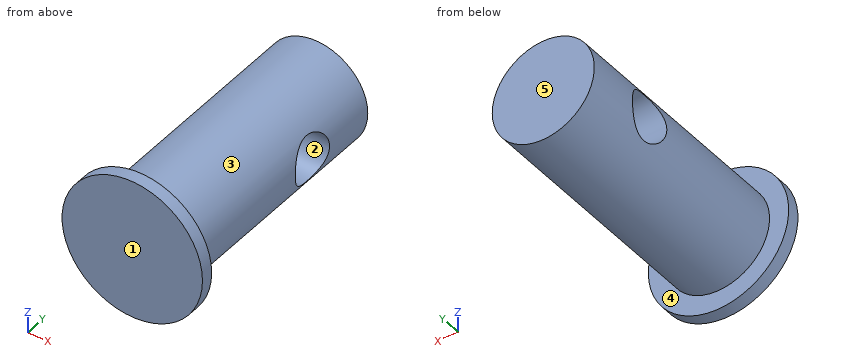
from build123d import *

# Parameters (mm, degrees)
SKETCH1_R           = 5.5
SKETCH1_R_2         = 4
BOSS_EXTRUDE1_DEPTH = 1
SKETCH1_2_R         = 4
BOSS_EXTRUDE2_DEPTH = 20
SKETCH2_R           = 1.8611768
CUT_EXTRUDE1_DEPTH  = 12


with BuildPart() as part:
    # Sketch1 → Boss-Extrude1 (new body)
    with BuildSketch(Plane(origin=(0, 0, 0), x_dir=(1, 0, 0), z_dir=(0, 1, 0))):
        Circle(SKETCH1_R)
        Circle(SKETCH1_R_2, mode=Mode.SUBTRACT)
    extrude(amount=BOSS_EXTRUDE1_DEPTH)

    # Sketch1<2> → Boss-Extrude2 (add)
    with BuildSketch(Plane(origin=(0, 0, 0), x_dir=(1, 0, 0), z_dir=(0, 1, 0))):
        Circle(SKETCH1_2_R)
    extrude(amount=BOSS_EXTRUDE2_DEPTH)

    # Sketch2 → Cut-Extrude1 (cut)
    with BuildSketch(Plane(origin=(4, 0, 0), x_dir=(0, 0, -1), z_dir=(1, 0, 0))):
        with Locations((0, 14)):
            Circle(SKETCH2_R)
    extrude(amount=-CUT_EXTRUDE1_DEPTH, mode=Mode.SUBTRACT)


solid = part.part
Work out the finished part from the listing and answer in its coordinate system (mm). Face numbers are marked on the shaded views. A direction names the side the tool comes from. Round coordinates to 2 decimals unless told otherwise and drop trailing zeros. Write each loop counter-clockwise with the first axis right and the second up, starting at its lowest first coordinate (ties: lowest second). Pieces come first, ordered by that corner, then holes. Notation, with made-up numbers: (-24.5, 27.25) - (-3.5, 27.25) arc R15 ccw to (-3.5, 56.25) - close; hole circle Ø5 at (16, -35.75). An arc over 180 degrees is marked (long way). Answer in a Markdown table with one row per item. Add a question column.
1. A cutting plane is placed at A-A, the plane z = 0. Determine the outline of the cut face in (x, y), and give its area (3 significant figures).
2. Given pin 1 (5 mm diameter, centred on x = 4, y = 6.5, fed in from -Z); pin 2 (2 mm diameter, centred on y = 12, z = 3.5, fed in from +X); pin 3 (3 mm diameter, centred on x = 0.5, y = 7.5, fed in from +Z); pin 4 (3 mm diameter, centred on x = 4, z = -3, fed in from +Y), each flat-ended and moving along its own axis, determine where each tip first touches the part or whether it passes through.
3. Find the intervals of material crossed by line 1 along Y through (x, z) = (2, 0); line 2 along Z through (x, y) = (0, 14); line 3 along Y through (x, z) = (-4.25, 1.5), in increasing order. Write a range as from..to.
4. A cutting plane is placed at D-D, the plane y = 4.5. Determine the outline of the cut face in (x, z).
5. A cutting plane is placed at C-C, the plane y = 14. Determine the outline of the cut face in (x, z).
6. A cutting plane is placed at B-B, the plane x = 0. Determine the outline of the cut face in (y, z), and give its area (3 significant figures).
7. For the marked faces 4 and 5, determine the directions among +Z, -Z, +X, -X, +Y, -Y from which every point of the face is accessible in a straight line to the end or side of a thin tool.
8. The mould has two halves that part along Z. Classify the marked faces 1, 2 and 3: +Z half, -Z half, draft (parallel to the pull), parting line (faces both ways), or undercut.
Worked out:
| question | item | result |
|---|---|---|
| 1 | outline | (-5.5, 0) - (5.5, 0) - (5.5, 1) - (4, 1) - (4, 12.14) - (-4, 12.14) - (-4, 1) - (-5.5, 1) - close; (-4, 15.86) - (4, 15.86) - (4, 20) - (-4, 20) - close |
| 1 | area | 133 mm^2 |
| 2 | pin 1 | z = -3.71 |
| 2 | pin 2 | x = 3.12 |
| 2 | pin 3 | z = 4 |
| 2 | pin 4 | y = 20 |
| 3 | line 1 | 0..12.14, 15.86..20 |
| 3 | line 2 | -4..-1.86, 1.86..4 |
| 3 | line 3 | 0..1 |
| 4 | outline | circle Ø8 at (0, 0) |
| 5 | outline | (-3.54, -1.86) arc R4 ccw to (3.54, -1.86) - close; (-3.54, 1.86) - (3.54, 1.86) arc R4 ccw to start |
| 6 | outline | (0, -5.5) - (1, -5.5) - (1, -4) - (20, -4) - (20, 4) - (1, 4) - (1, 5.5) - (0, 5.5) - close; hole circle Ø3.72 at (14, 0) |
| 6 | area | 152 mm^2 |
| 7 | face 4 | +Y |
| 7 | face 5 | +Z, -Z, +X, -X, +Y |
| 8 | face 1 | draft |
| 8 | face 2 | undercut |
| 8 | face 3 | parting line |
